Here's how the part is built. I have some questions about the finished solid (model axes, mm). A direction names the side the tool comes from. Round coordinates to 2 decimals unless told otherwise and drop trailing zeros. Loops run counter-clockwise (first coordinate to the right, second up) from the corner with the lowest first, then second, coordinate; pieces in that order, holes last. Notation, with made-up numbers: M -25,55 L -6,55 A24 ccw -6,79 Z; hole C -23.75,-7.5 d8. An arc over 180 degrees is marked long. Answer as a JSON object with one key per item and string values.
from build123d import *

# Parameters (mm, degrees)
F0_W           = 14.2875
F0_H           = 50.8
F2_R           = 7.0485
F3_DEPTH       = 88.901
F2_R_2         = 4.3815
F2_R_3         = 1.5875
F4_DEPTH       = 71.12
F6_DEPTH       = 28.576
F6_DEPTH_BACK  = 28.576
F7_R           = 4.3815
F8_DEPTH       = 15.24
F10_DEPTH      = 28.576
F10_DEPTH_BACK = 28.576
F11_R          = 2.517044934
F12_DEPTH      = 25.4


with BuildPart() as f1:
    # F0 (on Front) → F1 (revolve)
    with BuildSketch(Plane.XZ):
        Polygon((0, 88.9), (0, 50.8), (14.2875, 50.8), (28.575, 50.8), (28.575, 88.9), align=None)
        with Locations((7.14375, 25.4)):
            Rectangle(F0_W, F0_H)
    revolve(axis=Axis((0, 0, 25.4), (0, 0, 1)))

    # F2 (on face) → F3 (cut, through all)
    with BuildSketch(Plane(origin=(0, 0, 0), x_dir=(1, 0, 0), z_dir=(0, 0, -1))):
        with Locations((5.4483, 0)):
            Circle(F2_R)
    extrude(amount=-F3_DEPTH, mode=Mode.SUBTRACT)

    # F2 (on face) → F4 (cut)
    with BuildSketch(Plane(origin=(0, 0, 0), x_dir=(1, 0, 0), z_dir=(0, 0, -1))):
        with Locations((-8.1153, 0)):
            Circle(F2_R_2)
        with Locations((-3.3415136859, 7.1955672465)):
            Circle(F2_R_3)
    extrude(amount=-F4_DEPTH, mode=Mode.SUBTRACT)

    # F5 (on Front) → F6 (cut, two sides)
    with BuildSketch(Plane.XZ) as f6_sk:
        Polygon((-31.2208328396, 69.2149996758), (0, 92.5436764956), (-31.2208328396, 92.4983397126), align=None)
    extrude(amount=-F6_DEPTH, mode=Mode.SUBTRACT)
    extrude(f6_sk.sketch, amount=F6_DEPTH_BACK, mode=Mode.SUBTRACT)

    # F7 (on face) → F8 (cut)
    with BuildSketch(Plane(origin=(-44.3744352731, 0, 59.3864297025), x_dir=(0.8010695685, 0, 0.5985712543), z_dir=(-0.5985712543, 0, 0.8010695685))):
        with Locations((34.5289222896, 0)):
            Circle(F7_R)
    extrude(amount=-F8_DEPTH, mode=Mode.SUBTRACT)

    # F9 (on Right) → F10 (cut, two sides)
    with BuildSketch(Plane.YZ) as f10_sk:
        Polygon((-39.1586869955, 73.3165889978), (-11.2496605143, 92.7487313747), (-39.1586869955, 97.8193457674), align=None)
    extrude(amount=-F10_DEPTH, mode=Mode.SUBTRACT)
    extrude(f10_sk.sketch, amount=F10_DEPTH_BACK, mode=Mode.SUBTRACT)

    # F11 (on face) → F12 (cut)
    with BuildSketch(Plane(origin=(0, -47.1660624195, 67.7413153706), x_dir=(1, 0, 0), z_dir=(0, -0.5714046236, 0.8206684812))):
        with Locations((-4.5785461552, 30.4776653647)):
            Circle(F11_R)
    extrude(amount=-F12_DEPTH, mode=Mode.SUBTRACT)


solid = f1.part
Item 1: If we mould it in two halves opening along Y, with no side actions, what happens to faces 4 (the face through (-0.145, 4.289, 43.828)), 5 (the face through (12, 6, 88.9)), 6 (the face through (4.828, -22.759, 84.735)), 7 (the face through (27.255, 8.583, 65.883))? For each: pulls with the +Y half, pulls with the -Y half, needs draft (parallel to the pull), parting line crosses it, or undercut.
Resolved:
{"face 4": "undercut", "face 5": "needs draft", "face 6": "pulls with the -Y half", "face 7": "parting line crosses it"}
Item 2: Please list where these lines run through material, in increasing order: probe 1 along X at (y, z) = (-3.5, 34); probe 2 along X at (y, z) = (1.5, 49.5); probe 3 along Z at (x, y) = (24, 14.5). Write a range as from..to.
Resolved:
{"probe 1": "-13.85..-10.75, -5.48..-0.67, 11.57..13.85", "probe 2": "-14.21..-12.23, -4..-1.44, 12.34..14.21", "probe 3": "50.8..88.9"}
Item 3: I want a section at A-A, the plane y = 5.5. Please give me the cut outline in (x, z), then the cut area to 3 significant figures.
Resolved:
{"outline": "M -28.04,50.8 L -13.19,50.8 L -13.19,0 L 1.04,0 L 1.04,88.9 L -4.88,88.9 L -28.04,71.59 Z; M 9.86,0 L 13.19,0 L 13.19,50.8 L 28.04,50.8 L 28.04,88.9 L 9.86,88.9 Z", "area": "2,490 mm²"}
Item 4: I want a section at C-C, the plane y = -1. Please give me the cut outline in (x, z), then the cut area to 3 significant figures.
Resolved:
{"outline": "M -28.56,50.8 L -14.25,50.8 L -14.25,0 L -12.38,0 L -12.38,67.13 L -20.13,77.5 L -28.56,71.21 Z; M -13.3,82.61 L -4.71,71.12 L -3.85,71.12 L -3.85,0 L -1.53,0 L -1.53,88.9 L -4.88,88.9 Z; M 12.43,0 L 14.25,0 L 14.25,50.8 L 28.56,50.8 L 28.56,88.9 L 12.43,88.9 Z", "area": "1,470 mm²"}
Item 5: I want a section at B-B, the plane x = 0. Please give me the cut outline in (y, z) (1 decimal), then the cut area to 3 significant figures.
Resolved:
{"outline": "M -28.6,50.8 L -14.3,50.8 L -14.3,0 L -4.5,0 L -4.5,88.9 L -16.8,88.9 L -28.6,80.7 Z; M 4.5,0 L 14.3,0 L 14.3,50.8 L 28.6,50.8 L 28.6,88.9 L 4.5,88.9 Z", "area": "2,790 mm²"}
Item 6: I'm going to push flat-ended pins straight in: pin 1 Ø1 at (y, z) = (1.5, 33) entering from -X; pin 2 Ø4 at (x, z) = (-3.5, 21.5) entering from +Y; pin 3 Ø8 at (y, z) = (-4, 65) entering from -X (3 decimals); pin 4 Ø6 at (y, z) = (11, 58.5) entering from -X. Where does each tip first touch, or does it pass through?
Resolved:
{"pin 1": "x = -14.25", "pin 2": "y = 14.21", "pin 3": "x = -28.575", "pin 4": "x = -27.43"}
Item 7: I want a section at D-D, the plane y = 22.5. Please give me the cut outline in (x, z).
Resolved:
{"outline": "M -17.61,50.8 L 17.61,50.8 L 17.61,88.9 L -4.88,88.9 L -17.61,79.38 Z"}
Item 8: On a 3-axis mill with a long thin cutter (end or side, diameter ignored), from which of +Z, -Z, +X, -X, +Y, -Y can I reach the whole of each face in a straight line? I mean faces 1 (the face through (-3, 0, 0)), 2 (the face through (-14.274, 0.628, 25.756)), 3 (the face through (-5.22, -8.07, 64.01)). Say none if no direction works.
Resolved:
{"face 1": "-Z, +X, -X, +Y, -Y", "face 2": "-Z", "face 3": "none"}
